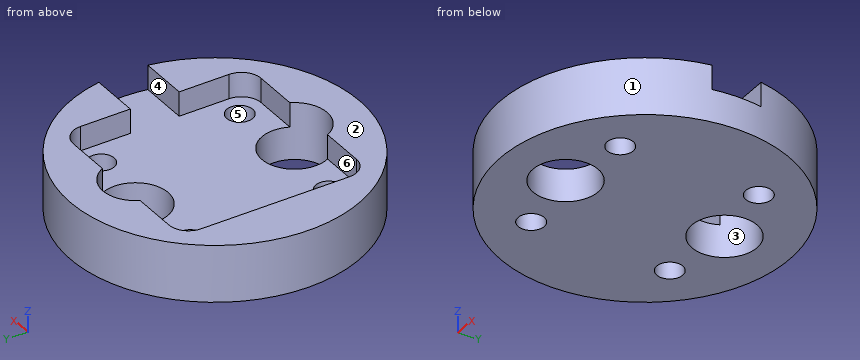
```python
from build123d import *

# Parameters (mm, degrees)
SKETCH1_R           = 17.75
SKETCH1_R_2         = 4
BOSS_EXTRUDE1_DEPTH = 7
CUT_EXTRUDE1_START  = 7
SKETCH1_3_W         = 23
SKETCH1_3_H         = 23
SKETCH1_3_R         = 1.6
CUT_EXTRUDE1_DEPTH  = 3
SKETCH1_4_R         = 1.6
CUT_EXTRUDE3_DEPTH  = 27.060026861
CUT_EXTRUDE4_START  = -3
CUT_EXTRUDE4_DEPTH  = 3
FILLET1_R           = 2.4


with BuildPart() as part:
    # Sketch1 → Boss-Extrude1 (new body)
    with BuildSketch(Plane(origin=(0, 0, 0), x_dir=(0, 1, 0), z_dir=(0, 0, 1))):
        with Locations(Location((0, 0, 0), (0, 0, 270))):
            Circle(SKETCH1_R)
        with Locations(Location((9.75, 0, 0), (0, 0, 270))):
            Circle(SKETCH1_R_2, mode=Mode.SUBTRACT)
        with Locations(Location((-9.75, 0, 0), (0, 0, 270))):
            Circle(SKETCH1_R_2, mode=Mode.SUBTRACT)
    extrude(amount=BOSS_EXTRUDE1_DEPTH)

    # Sketch1<3> → Cut-Extrude1 (cut)
    # profile 1 of 5: a face of its own
    with BuildSketch(Plane(origin=(0, 0, 0), x_dir=(0, 1, 0), z_dir=(0, 0, 1)).offset(CUT_EXTRUDE1_START)):
        Rectangle(SKETCH1_3_W, SKETCH1_3_H)
        with Locations((-8.5, -8.5)):
            Circle(SKETCH1_3_R, mode=Mode.SUBTRACT)
        with Locations((8.5, -8.5)):
            Circle(SKETCH1_3_R, mode=Mode.SUBTRACT)
        with Locations((8.5, 8.5)):
            Circle(SKETCH1_3_R, mode=Mode.SUBTRACT)
        with Locations((-8.5, 8.5)):
            Circle(SKETCH1_3_R, mode=Mode.SUBTRACT)
    # profile 2 of 5: a face of its own
    with BuildSketch(Plane(origin=(0, 0, 0), x_dir=(0, 1, 0), z_dir=(0, 0, 1)).offset(CUT_EXTRUDE1_START)):
        with Locations((-8.5, 8.5)):
            Circle(SKETCH1_3_R)
    # profile 3 of 5: a face of its own
    with BuildSketch(Plane(origin=(0, 0, 0), x_dir=(0, 1, 0), z_dir=(0, 0, 1)).offset(CUT_EXTRUDE1_START)):
        with Locations((8.5, 8.5)):
            Circle(SKETCH1_3_R)
    # profile 4 of 5: a face of its own
    with BuildSketch(Plane(origin=(0, 0, 0), x_dir=(0, 1, 0), z_dir=(0, 0, 1)).offset(CUT_EXTRUDE1_START)):
        with Locations((-8.5, -8.5)):
            Circle(SKETCH1_3_R)
    # profile 5 of 5: a face of its own
    with BuildSketch(Plane(origin=(0, 0, 0), x_dir=(0, 1, 0), z_dir=(0, 0, 1)).offset(CUT_EXTRUDE1_START)):
        with Locations((8.5, -8.5)):
            Circle(SKETCH1_3_R)
    extrude(amount=-CUT_EXTRUDE1_DEPTH, mode=Mode.SUBTRACT)

    # Sketch1<4> → Cut-Extrude3 (cut, through all)
    with BuildSketch(Plane(origin=(0, 0, 0), x_dir=(0, 1, 0), z_dir=(0, 0, 1))):
        with Locations(Location((-8.5, -8.5, 0), (0, 0, 270))):
            Circle(SKETCH1_4_R)
        with Locations(Location((8.5, -8.5, 0), (0, 0, 270))):
            Circle(SKETCH1_4_R)
        with Locations(Location((8.5, 8.5, 0), (0, 0, 270))):
            Circle(SKETCH1_4_R)
        with Locations(Location((-8.5, 8.5, 0), (0, 0, 270))):
            Circle(SKETCH1_4_R)
    extrude(amount=CUT_EXTRUDE3_DEPTH, mode=Mode.SUBTRACT)

    # Sketch2 → Cut-Extrude4 (cut)
    with BuildSketch(Plane.XY.offset(7).offset(CUT_EXTRUDE4_START)):
        with BuildLine():
            Line((11.5, 3), (17.494642037, 3))
            ThreePointArc((17.494642037, 3), (17.75, 0), (17.494642037, -3))
            Line((17.494642037, -3), (11.5, -3))
            Line((11.5, -3), (11.5, 3))
        make_face()
    extrude(amount=CUT_EXTRUDE4_DEPTH, mode=Mode.SUBTRACT)

    # Fillet1
    fillet1_edges = [part.edges().sort_by_distance(p)[0] for p in [
        (-11.5, -11.5, 5.5),
        (-11.5, 11.5, 5.5),
        (11.5, 11.5, 5.5),
        (11.5, -11.5, 5.5),
    ]]
    fillet(fillet1_edges, radius=FILLET1_R)


solid = part.part
```
Part model, mm, in its own coordinate system. Face numbers are marked on the shaded views. A direction names the side the tool comes from. Round coordinates to 2 decimals unless told otherwise and drop trailing zeros. Write each loop counter-clockwise with the first axis right and the second up, starting at its lowest first coordinate (ties: lowest second). Pieces come first, ordered by that corner, then holes. Notation, with made-up numbers: M -35,9 L -3,9 A33 cw -3,47 Z; hole C -6,55.5 d11. An arc over 180 degrees is marked long. Answer as CSV lines item,"result". Start each with the question number.
1) Band-saw the part on C-C (y = -7.5). List the corners of the cut face in (x, z), then the cut area to 3 significant figures.
2) Band-saw the part on B-B (x = 0). List the corners of the cut face in (y, z).
3) Band-saw the part on A-A (z = 1.5). List the corners of the cut face in (x, y).
4) Which spindle directions (+Z, -Z, +X, -X, +Y, -Y) get a long thin tool onto all of the face, cutting with end or side? Do the marked faces 4, 5 and 6. Say none if no direction does.
5) Drill centre lines: L1, parallel to Y at x = 0, z = 3.5; L2, parallel to Y at x = 0, z = 4.75; L3, parallel to X at y = -8.5, z = 3. Where is each one in solid material? Low to high.
6) Band-saw the part on D-D (y = 0). List the corners of the cut face in (x, z).
7) Drop flat-ended pins along their axis: pin 1 (3.5 mm diameter, centred on x = 5.5, z = 5.5, fed in from -Y); pin 2 (1.5 mm diameter, centred on x = -0.5, z = 3.5, fed in from -Y); pin 3 (2.5 mm diameter, centred on x = 15, z = 5.5, fed in from +Y) (3 decimals); pin 4 (0.9 mm diameter, centred on y = -5, z = 5.5, fed in from -X). Give the stop position or say it passes through.
8) Mould opens along X. For the marked faces 1, 2 and 3 say: +X half, -X half, draft (parallel to the pull), parting line (faces both ways), or undercut.
Worked out:
1,outline,"M -16.09,0 L -9.75,0 L -9.75,4 L -11.5,4 L -11.5,7 L -16.09,7 Z; M -7.25,0 L -3.31,0 L -3.31,4 L -7.25,4 Z; M 3.31,0 L 7.25,0 L 7.25,4 L 3.31,4 Z; M 9.75,0 L 16.09,0 L 16.09,7 L 11.5,7 L 11.5,4 L 9.75,4 Z"
1,area,"110 mm²"
2,outline,"M -17.75,0 L -13.75,0 L -13.75,7 L -17.75,7 Z; M -5.75,0 L 5.75,0 L 5.75,4 L -5.75,4 Z; M 13.75,0 L 17.75,0 L 17.75,7 L 13.75,7 Z"
3,outline,"C 0,0 d35.5; hole C -8.5,-8.5 d3.2; hole C -8.5,8.5 d3.2; hole C 0,-9.75 d8; hole C 0,9.75 d8; hole C 8.5,-8.5 d3.2; hole C 8.5,8.5 d3.2"
4,face 4,"+Z, +X"
4,face 5,"+Z, -Z"
4,face 6,"+Z"
5,L1,"-17.75 to -13.75, -5.75 to 5.75, 13.75 to 17.75"
5,L2,"-17.75 to -13.75, 13.75 to 17.75"
5,L3,"-15.58 to -10.1, -6.9 to -3.8, 3.8 to 6.9, 10.1 to 15.58"
6,outline,"M -17.75,0 L 17.75,0 L 17.75,4 L -11.5,4 L -11.5,7 L -17.75,7 Z"
7,pin 1,"y = -17.35"
7,pin 2,"y = -17.75"
7,pin 3,"y = 11.225"
7,pin 4,"x = -17.16"
8,face 1,"parting line"
8,face 2,"draft"
8,face 3,"undercut"
